Geometry check sheet. Reference: the model listing, model coordinates, mm. Face numbers are marked on the shaded views. A direction names the side the tool comes from. Give positions to 0.01 mm unless a question says otherwise; leave off trailing zeros. Order: outer loops, then holes, each group sorted by start corner. A loop starts at its lowest first (then second) coordinate and runs counter-clockwise, first axis right, second up. Notation, with made-up numbers: M 34.25,19.25 L 89.25,19.25 A25 ccw 89.25,45.25 Z; hole C -6,82.5 d5. An arc over 180 degrees is marked long. Answer as CSV lines item,"result".
from build123d import *

# Parameters (mm, degrees)
SKETCH1_R           = 277.5
BOSS_EXTRUDE1_DEPTH = 10
SKETCH2_W           = 400
SKETCH2_H           = 400
BOSS_EXTRUDE2_DEPTH = 50
FILLET1_R           = 50
SKETCH3_R           = 130
BOSS_EXTRUDE3_DEPTH = 200


with BuildPart() as part:
    # Sketch1 → Boss-Extrude1 (new body)
    with BuildSketch(Plane(origin=(0, 0, 0), x_dir=(1, 0, 0), z_dir=(0, 1, 0))):
        with Locations(Location((0, 0, 0), (0, 0, 270))):
            Circle(SKETCH1_R)
    extrude(amount=BOSS_EXTRUDE1_DEPTH)

    # Sketch2 → Boss-Extrude2 (add)
    with BuildSketch(Plane(origin=(0, 10, 0), x_dir=(1, 0, 0), z_dir=(0, 1, 0))):
        with Locations((0.651230283, 0)):
            Rectangle(SKETCH2_W, SKETCH2_H)
    extrude(amount=BOSS_EXTRUDE2_DEPTH)

    # Fillet1
    # the kernel refuses this fillet: 50 mm, written as the material it takes off along each edge
    with BuildSketch(Plane(origin=(200.651230283, 10, 200), x_dir=(-1, 0, 0), z_dir=(0, 1, 0))) as fillet1_piece_1:
        with BuildLine():
            CenterArc((FILLET1_R, -FILLET1_R), FILLET1_R, 90, 90)
            Line((0, -FILLET1_R), (0, 0))
            Line((0, 0), (FILLET1_R, 0))
        make_face()
    extrude(amount=175, mode=Mode.SUBTRACT)
    with BuildSketch(Plane(origin=(200.651230283, 10, -200), x_dir=(-1, 0, 0), z_dir=(0, 1, 0)), Plane(origin=(-199.348769717, 10, -200), x_dir=(0, 0, 1), z_dir=(0, 1, 0)), Plane(origin=(-199.348769717, 10, 200), x_dir=(1, 0, 0), z_dir=(0, 1, 0))) as fillet1_piece_2:
        with BuildLine():
            CenterArc((FILLET1_R, FILLET1_R), FILLET1_R, 180, 90)
            Line((0, FILLET1_R), (0, 0))
            Line((0, 0), (FILLET1_R, 0))
        make_face()
    extrude(amount=175, mode=Mode.SUBTRACT)

    # Sketch3 → Boss-Extrude3 (add)
    with BuildSketch(Plane(origin=(0, 60, 0), x_dir=(1, 0, 0), z_dir=(0, 1, 0))):
        with Locations(Location((0, 0, 0), (0, 0, 270))):
            Circle(SKETCH3_R)
    extrude(amount=BOSS_EXTRUDE3_DEPTH)


solid = part.part
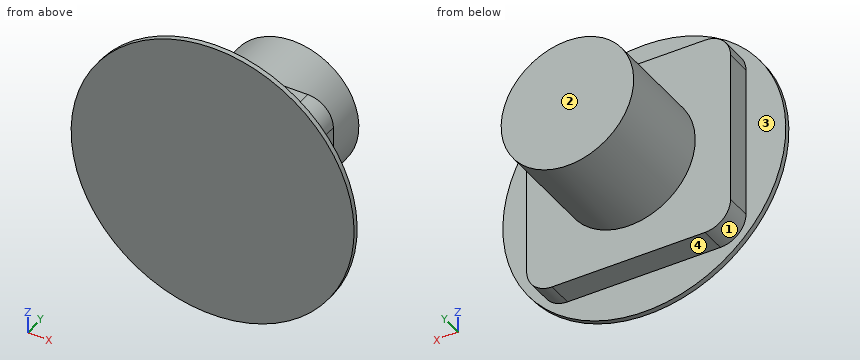
(1) Section check A-A on z = 0. Enter the section's corners in (x, y), then the cut area to 4 significant figures.
The answers:
outline,"M -277.5,0 L 277.5,0 L 277.5,10 L 200.65,10 L 200.65,60 L 130,60 L 130,260 L -130,260 L -130,60 L -199.35,60 L -199.35,10 L -277.5,10 Z"
area,"77,550 mm2"
(2) Material ranges on line 1 (Y direction, x = -148, z = -31.5); line 2 (X direction, y = 39, z = 89.5); line 3 (Y direction, x = -90, z = 201.5), recorded low to high.
The answers:
line 1,"y = 0 to 60"
line 2,"x = -199.35 to 200.65"
line 3,"y = 0 to 10"
(3) Section check B-B on y = 40. Enter the section's corners in (x, z).
The answers:
outline,"M -199.35,-150 A50 ccw -149.35,-200 L 150.65,-200 A50 ccw 200.65,-150 L 200.65,150 A50 ccw 150.65,200 L -149.35,200 A50 ccw -199.35,150 Z"
(4) Tool access check on the marked faces 1, 2, 3 and 4. Record the directions out of +Z, -Z, +X, -X, +Y, -Y that give a thin tool (end or side, any length) a straight path to the whole face; none if there is none.
The answers:
face 1,"-Z, -X, +Y"
face 2,"+Z, -Z, +X, -X, +Y"
face 3,"+Y"
face 4,"-Z, +X, -X, +Y"
(5) Section check C-C on x = 0. Enter the section's corners in (y, z).
The answers:
outline,"M 0,-277.5 L 10,-277.5 L 10,-200 L 60,-200 L 60,-130 L 260,-130 L 260,130 L 60,130 L 60,200 L 10,200 L 10,277.5 L 0,277.5 Z"
(6) Gauge pin test, flat ends, axial feed: P1, Ø1.5, axis at y = 150.5, z = -37, coming from the +X side; P2, Ø10, axis at x = 41.5, z = -153.5, coming from the +Y side; P3, Ø25, axis at y = 42.5, z = 65, coming from the +X side. Record the tip position at first contact, or that the pin passes through.
The answers:
P1,"stops at x = 124.84"
P2,"stops at y = 60"
P3,"stops at x = 200.65"
(7) Section check D-D on z = -193. Enter the section's corners in (x, y), then the cut area to 3 significant figures.
The answers:
outline,"M -199.39,0 L 199.39,0 L 199.39,10 L 176.17,10 L 176.17,60 L -174.86,60 L -174.86,10 L -199.39,10 Z"
area,"21,500 mm2"
